```python
from build123d import *

# Parameters (mm, degrees)
SKETCH3_R                = 43.942
BOSS_EXTRUDE1_DEPTH      = 15.24
BOSS_EXTRUDE2_REACH      = 2235.699
BOSS_EXTRUDE2_END_RADIUS = 78.32293196
SKETCH4_W                = 3.175
SKETCH4_H                = 203.2
CUT_EXTRUDE1_REACH       = 2225.452
FILLET1_R                = 2.54
CIRPATTERN1_COUNT        = 4
FILLET1_OF_CIRPATTERN1_R = 2.54


with BuildPart() as part:
    # Sketch2 → Revolve1 (revolve)
    with BuildSketch(Plane(origin=(0, 0, 0), x_dir=(0, 0, -1), z_dir=(1, 0, 0))):
        with BuildLine():
            Line((156.718, 78.322932), (2192.2105, 78.322932))
            Line((2192.2105, 78.322932), (2192.2105, 4e-08))
            Line((2192.2105, 4e-08), (4.964740615, 4e-08))
            ThreePointArc((4.964740615, 4e-08), (5.897622526, 4.522765989), (8.543990278, 8.307263076))
            add(Edge.make_bspline(
                [(8.543990278, 8.307263076), (82.630995139, 78.322932), (156.718, 78.322932)],
                knots=[0.068626342, 0.068626342, 0.068626342, 0.915329667, 0.915329667, 0.915329667], degree=2))
        make_face()
    revolve(axis=Axis((0, 4e-08, -2192.2105), (0, 0, 1)))

    # Sketch3 → Boss-Extrude1 (add)
    with BuildSketch(Plane(origin=(0, 0, -2192.2105), x_dir=(-1, 0, 0), z_dir=(0, 0, -1))):
        with Locations(Location((0, 0, 0), (0, 0, 270))):
            Circle(SKETCH3_R)
    extrude(amount=BOSS_EXTRUDE1_DEPTH)

    # Boss-Extrude2: up to this cylinder (the profile starts outside it)
    boss_extrude2_end = Plane(origin=(0, 4e-08, -2087.4355), z_dir=(0, 0, -1)) * Cylinder(BOSS_EXTRUDE2_END_RADIUS, 4629.043863919, mode=Mode.PRIVATE)
    # Sketch4 → Boss-Extrude2 (add, up to the surface)
    with BuildSketch(Plane(origin=(0, 254, 0), x_dir=(1, 0, 0), z_dir=(0, 1, 0)), mode=Mode.PRIVATE) as boss_extrude2_sk1:
        with Locations((0, 2087.4355)):
            Rectangle(SKETCH4_W, SKETCH4_H)
    boss_extrude2_tool1 = extrude(boss_extrude2_sk1.sketch, amount=-BOSS_EXTRUDE2_REACH, mode=Mode.PRIVATE) - boss_extrude2_end
    boss_extrude2 = boss_extrude2_tool1.solids().sort_by_distance((0, 254, -2087.4355))[0]
    add(boss_extrude2)

    # Sketch5 → Cut-Extrude1 (cut, up to next)
    with BuildSketch(Plane.ZY.offset(1.5875), mode=Mode.PRIVATE) as cut_extrude1_sk1:
        Polygon((-2189.0355, 224.356842107), (-2087.4355, 224.356842107), (-1985.8355, 78.306842107), (-1985.8355, 254), (-2189.0355, 254), align=None)
    cut_extrude1_tool1 = extrude(cut_extrude1_sk1.sketch, amount=-CUT_EXTRUDE1_REACH, mode=Mode.PRIVATE) & part.part
    cut_extrude1 = cut_extrude1_tool1.solids().sort_by_distance((-1.5875, 204.128915, -2050.052252))[0]
    add(cut_extrude1, mode=Mode.SUBTRACT)

    # Fillet1
    # the kernel refuses this fillet: 2.54 mm, written as the material it adds along each edge
    with BuildSketch(Plane(origin=(-1.5875, 78.306842107, -1979.708797857), x_dir=(-0.9993639751492599, -0.03566013423796214, 0), z_dir=(0, 0, -1))) as fillet1_piece_1_section:
        with BuildLine():
            CenterArc((2.450992889, 2.539698904), FILLET1_R, 182.043608469, 87.074170623)
            Line((-0.087391608, 2.449122163), (0, 0))
            ThreePointArc((0, 0), (1.205942189, 0.009284527), (2.411884379, 0))
        make_face()
    fillet1_piece_1 = extrude(amount=209.326702143, mode=Mode.PRIVATE)
    fillet1_piece_1 = split(fillet1_piece_1, bisect_by=Plane(origin=(-3.095055571, 78.248638535, -1985.795010558), z_dir=(0, -0.5710644881985977, -0.8209052017854886)), keep=Keep.TOP, mode=Mode.PRIVATE)
    add(fillet1_piece_1)
    with BuildSketch(Plane(origin=(1.5875, 78.306842107, -1979.708797857), x_dir=(0.9993639751492599, -0.035660134237962375, 0), z_dir=(0, 0, -1))) as fillet1_piece_2_section:
        with BuildLine():
            CenterArc((2.450992889, -2.539698904), FILLET1_R, 90.882220908, 87.074170623)
            Line((-0.087391608, -2.449122163), (0, 0))
            ThreePointArc((0, 0), (1.205942189, -0.009284527), (2.411884379, 0))
        make_face()
    fillet1_piece_2 = extrude(amount=209.326702143, mode=Mode.PRIVATE)
    fillet1_piece_2 = split(fillet1_piece_2, bisect_by=Plane(origin=(3.095055571, 78.248638535, -1985.795010558), z_dir=(0, -0.5710644881985977, -0.8209052017854886)), keep=Keep.TOP, mode=Mode.PRIVATE)
    add(fillet1_piece_2)

    # CirPattern1: Boss-Extrude2, Cut-Extrude1 ×4 about axis
    cirpattern1_axis = Axis((0, 1.7e-08, 0), (0, 0, 1))
    add([boss_extrude2.rotate(cirpattern1_axis, i * 360 / CIRPATTERN1_COUNT) for i in range(1, CIRPATTERN1_COUNT)])
    add([cut_extrude1.rotate(cirpattern1_axis, i * 360 / CIRPATTERN1_COUNT) for i in range(1, CIRPATTERN1_COUNT)], mode=Mode.SUBTRACT)

    # Fillet1 of CirPattern1
    # the kernel refuses this fillet: 2.54 mm, written as the material it adds along each edge
    with BuildSketch(Plane(origin=(-78.306842067, -1.587499983, -1979.708797917), x_dir=(0.03566013452716192, -0.9993639751389404, 0), z_dir=(0, 0, -1))) as fillet1_of_cirpattern1_piece_1_section:
        with BuildLine():
            CenterArc((2.450992888, 2.539698904), FILLET1_OF_CIRPATTERN1_R, 182.043608486, 87.074170607)
            Line((-0.087391609, 2.449122163), (0, 0))
            ThreePointArc((0, 0), (1.205942189, 0.009284527), (2.411884378, 0))
        make_face()
    fillet1_of_cirpattern1_piece_1 = extrude(amount=209.326702083, mode=Mode.PRIVATE)
    fillet1_of_cirpattern1_piece_1 = split(fillet1_of_cirpattern1_piece_1, bisect_by=Plane(origin=(-78.248638505, -3.095055439, -1985.79501055), z_dir=(0.5710644881985977, 0, -0.8209052017854886)), keep=Keep.TOP, mode=Mode.PRIVATE)
    add(fillet1_of_cirpattern1_piece_1)
    with BuildSketch(Plane(origin=(-78.306842068, 1.587500017, -1979.708797911), x_dir=(0.03566013394875642, 0.9993639751595796, 0), z_dir=(0, 0, -1))) as fillet1_of_cirpattern1_piece_2_section:
        with BuildLine():
            CenterArc((2.450992889, -2.539698904), FILLET1_OF_CIRPATTERN1_R, 90.882220908, 87.074170639)
            Line((-0.087391608, -2.449122164), (0, 0))
            ThreePointArc((0, 0), (1.20594219, -0.009284527), (2.411884379, 0))
        make_face()
    fillet1_of_cirpattern1_piece_2 = extrude(amount=209.326702089, mode=Mode.PRIVATE)
    fillet1_of_cirpattern1_piece_2 = split(fillet1_of_cirpattern1_piece_2, bisect_by=Plane(origin=(-78.248638506, 3.095055478, -1985.79501055), z_dir=(0.5710644881985977, 0, -0.8209052017854886)), keep=Keep.TOP, mode=Mode.PRIVATE)
    add(fillet1_of_cirpattern1_piece_2)
    with BuildSketch(Plane(origin=(1.5875, -78.306842027, -1979.708797972), x_dir=(0.9993639751492599, 0.03566013423796238, 0), z_dir=(0, 0, -1))) as fillet1_of_cirpattern1_piece_3_section:
        with BuildLine():
            CenterArc((2.450992889, 2.539698904), FILLET1_OF_CIRPATTERN1_R, 182.043608469, 87.074170623)
            Line((-0.087391608, 2.449122163), (0, 0))
            ThreePointArc((0, 0), (1.205942189, 0.009284527), (2.411884379, 0))
        make_face()
    fillet1_of_cirpattern1_piece_3 = extrude(amount=209.326702028, mode=Mode.PRIVATE)
    fillet1_of_cirpattern1_piece_3 = split(fillet1_of_cirpattern1_piece_3, bisect_by=Plane(origin=(3.095055347, -78.248638477, -1985.795010542), z_dir=(0, 0.5710644881985977, -0.8209052017854886)), keep=Keep.TOP, mode=Mode.PRIVATE)
    add(fillet1_of_cirpattern1_piece_3)
    with BuildSketch(Plane(origin=(-1.5875, -78.306842027, -1979.708797972), x_dir=(-0.9993639751492599, 0.03566013423796186, 0), z_dir=(0, 0, -1))) as fillet1_of_cirpattern1_piece_4_section:
        with BuildLine():
            CenterArc((2.450992889, -2.539698904), FILLET1_OF_CIRPATTERN1_R, 90.882220908, 87.074170623)
            Line((-0.087391608, -2.449122163), (0, 0))
            ThreePointArc((0, 0), (1.205942189, -0.009284527), (2.411884379, 0))
        make_face()
    fillet1_of_cirpattern1_piece_4 = extrude(amount=209.326702028, mode=Mode.PRIVATE)
    fillet1_of_cirpattern1_piece_4 = split(fillet1_of_cirpattern1_piece_4, bisect_by=Plane(origin=(-3.095055347, -78.248638477, -1985.795010542), z_dir=(0, 0.5710644881985977, -0.8209052017854886)), keep=Keep.TOP, mode=Mode.PRIVATE)
    add(fillet1_of_cirpattern1_piece_4)
    with BuildSketch(Plane(origin=(78.306842068, 1.587500017, -1979.708797911), x_dir=(-0.03566013394876229, 0.9993639751595792, 0), z_dir=(0, 0, -1))) as fillet1_of_cirpattern1_piece_5_section:
        with BuildLine():
            CenterArc((2.450992889, 2.539698904), FILLET1_OF_CIRPATTERN1_R, 182.043608452, 87.074170639)
            Line((-0.087391608, 2.449122164), (0, 0))
            ThreePointArc((0, 0), (1.20594219, 0.009284527), (2.411884379, 0))
        make_face()
    fillet1_of_cirpattern1_piece_5 = extrude(amount=209.326702089, mode=Mode.PRIVATE)
    fillet1_of_cirpattern1_piece_5 = split(fillet1_of_cirpattern1_piece_5, bisect_by=Plane(origin=(78.248638506, 3.095055478, -1985.79501055), z_dir=(-0.5710644881985977, 0, -0.8209052017854886)), keep=Keep.TOP, mode=Mode.PRIVATE)
    add(fillet1_of_cirpattern1_piece_5)
    with BuildSketch(Plane(origin=(78.306842067, -1.587499983, -1979.708797917), x_dir=(-0.03566013452716244, -0.9993639751389404, 0), z_dir=(0, 0, -1))) as fillet1_of_cirpattern1_piece_6_section:
        with BuildLine():
            CenterArc((2.450992888, -2.539698904), FILLET1_OF_CIRPATTERN1_R, 90.882220908, 87.074170607)
            Line((-0.087391609, -2.449122163), (0, 0))
            ThreePointArc((0, 0), (1.205942189, -0.009284527), (2.411884378, 0))
        make_face()
    fillet1_of_cirpattern1_piece_6 = extrude(amount=209.326702083, mode=Mode.PRIVATE)
    fillet1_of_cirpattern1_piece_6 = split(fillet1_of_cirpattern1_piece_6, bisect_by=Plane(origin=(78.248638505, -3.095055439, -1985.79501055), z_dir=(-0.5710644881985977, 0, -0.8209052017854886)), keep=Keep.TOP, mode=Mode.PRIVATE)
    add(fillet1_of_cirpattern1_piece_6)


solid = part.part
```
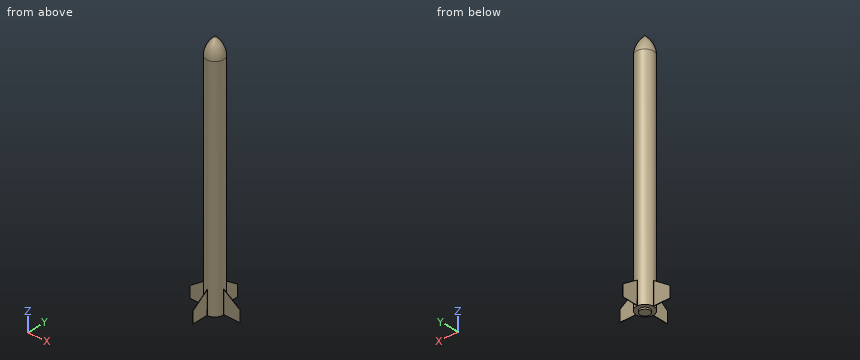
Model file for the job. Use its own axes, mm. Give positions to 0.01 mm unless a question says otherwise; leave off trailing zeros. Write each loop counter-clockwise with the first axis right and the second up, starting at its lowest first coordinate (ties: lowest second). Pieces come first, ordered by that corner, then holes. Notation, with made-up numbers: (67.5, 35.25) - (123.5, 35.25) arc R18 cw to (123.5, 70.25) - close; hole circle Ø8 at (52, 22). An arc over 180 degrees is marked (long way). One line per question, with ' | ' between items. Start each with the question number.
(1) Slice it at B-B on y = 154.5. Write the cut outline in (x, z).
(2) Pin check, flat tips, straight feed: P1, Ø2, axis at y = -52, z = -1941, coming from the +X side; P2, Ø8, axis at y = 18.5, z = -1421.5, coming from the +X side; P3, Ø4, axis at x = -48, z = -963, coming from the -Y side. Stop position of each tip, or through.
(3) Wall check: line 1 along Y through (x, z) = (176, -2112.5); line 2 along X through (y, z) = (6.5, -537); line 3 along Z through (x, y) = (-2, 54.5). Give the ranges that are in metal, low to high. Write a range as from..to.
(4) Slice it at A-A on z = -2023.5. Write the cut outline in (x, y), plus the area to 3 significant figures.
(5) Slice it at C-C on z = -502. Write the cut outline in (x, y).
Results below:
1) outline: (-1.59, -2189.04) - (1.59, -2189.04) - (1.59, -2038.84) - (-1.59, -2038.84) - close
2) P1: x = 59.44 | P2: x = 76.97 | P3: y = -63.39
3) line 1: -1.59..1.59 | line 2: -78.05..78.05 | line 3: -2192.21..-70.35
4) outline: (-132.45, -1.59) - (-80.76, -1.59) arc R2.54 cw to (-78.22, -4) arc R78.32 ccw to (-4, -78.22) arc R2.54 cw to (-1.59, -80.76) - (-1.59, -132.45) - (1.59, -132.45) - (1.59, -80.76) arc R2.54 cw to (4, -78.22) arc R78.32 ccw to (78.22, -4) arc R2.54 cw to (80.76, -1.59) - (132.45, -1.59) - (132.45, 1.59) - (80.76, 1.59) arc R2.54 cw to (78.22, 4) arc R78.32 ccw to (4, 78.22) arc R2.54 cw to (1.59, 80.76) - (1.59, 132.45) - (-1.59, 132.45) - (-1.59, 80.76) arc R2.54 cw to (-4, 78.22) arc R78.32 ccw to (-78.22, 4) arc R2.54 cw to (-80.76, 1.59) - (-132.45, 1.59) - close | area: 20,000 mm^2
5) outline: circle Ø156.65 at (0, 0)
